```python
from build123d import *

# Parameters (mm, degrees)
SKETCH_1_W      = 99
SKETCH_1_H      = 29
EXTRUDE_2_DEPTH = 2
FILLET_1_R      = 2.5
SKETCH_3_W      = 103
SKETCH_3_H      = 33
EXTRUDE_3_DEPTH = 1
FILLET_2_R      = 0.2


with BuildPart() as part:
    # Эскиз1 → Бобышка-Вытянуть2 (new body)
    with BuildSketch(Plane.XY):
        with Locations((-70, 10)):
            Rectangle(SKETCH_1_W, SKETCH_1_H)
    extrude(amount=-EXTRUDE_2_DEPTH)

    # Скругление1
    fillet_1_edges = [part.edges().sort_by_distance(p)[0] for p in [
        (-119.5, 24.5, -1),
        (-20.5, 24.5, -1),
        (-20.5, -4.5, -1),
        (-119.5, -4.5, -1),
    ]]
    fillet(fillet_1_edges, radius=FILLET_1_R)

    # Эскиз3 → Бобышка-Вытянуть3 (add)
    with BuildSketch(Plane.XY.offset(-2)):
        with Locations((-70, 10)):
            Rectangle(SKETCH_3_W, SKETCH_3_H)
    extrude(amount=-EXTRUDE_3_DEPTH)

    # Скругление2
    fillet_2_edges = [part.edges().sort_by_distance(p)[0] for p in [
        (-70, -4.5, 0),
        (-119.5, 10, 0),
        (-20.5, 10, 0),
        (-70, 24.5, 0),
        (-21.232233047, 23.767766953, 0),
        (-118.767766953, 23.767766953, 0),
        (-118.767766953, -3.767766953, 0),
        (-21.232233047, -3.767766953, 0),
    ]]
    fillet(fillet_2_edges, radius=FILLET_2_R)


solid = part.part
```
Here's how the part is built. I have some questions about the finished solid (model axes, mm). A direction names the side the tool comes from. Coordinates: 2 decimals unless noted, no trailing zeros. Loops run counter-clockwise (first coordinate to the right, second up) from the corner with the lowest first, then second, coordinate; pieces in that order, holes last. Notation, with made-up numbers: M 68.5,-37.5 L 95.5,-37.5 A34 cw 95.5,-3.5 Z; hole C 52,-27 d4. An arc over 180 degrees is marked long. One line per item, written item: value.
1. Imagine slicing it at A-A (y = 16.5). List the corners of the cut face in (x, z) for me.
Geometry says:
outline: M -121.5,-3 L -18.5,-3 L -18.5,-2 L -20.5,-2 L -20.5,-0.2 A0.2 ccw -20.7,0 L -119.3,0 A0.2 ccw -119.5,-0.2 L -119.5,-2 L -121.5,-2 Z
2. Please list where these lines run through material, in increasing order: probe 1 along Y at (x, z) = (-61, -0.15); probe 2 along X at (y, z) = (20, -0.5).
Geometry says:
probe 1: y = -4.49 to 24.49
probe 2: x = -119.5 to -20.5
3. On a 3-axis mill with a long thin cutter (end or side, diameter ignored), from which of +Z, -Z, +X, -X, +Y, -Y can I reach the whole of each face in a straight line? I mean faces 1 (the flat face through (-71, 24.5, -1)), 2 (the flat face through (-119.5, 10, -1)), 3 (the cylindrical face through (-118.787, 23.748, -1.113)). Say none if no direction works.
Geometry says:
face 1: +Z, +X, -X, +Y
face 2: +Z, -X, +Y, -Y
face 3: +Z, -X, +Y
4. Will these pins go through, and if not, where does the flat tip stop? pin 1 Ø1.4 at (x, z) = (-65, -1) entering from -Y; pin 2 Ø0.5 at (x, z) = (-54.5, -1) entering from +Y; pin 3 Ø0.9 at (y, z) = (15, -1.5) entering from -X.
Geometry says:
pin 1: stops at y = -4.5
pin 2: stops at y = 24.5
pin 3: stops at x = -119.5
5. Imagine slicing it at B-B (z = -1.45). List the corners of the cut face in (x, y) for me, and give its area (3 significant figures).
Geometry says:
outline: M -119.5,-2 A2.5 ccw -117,-4.5 L -23,-4.5 A2.5 ccw -20.5,-2 L -20.5,22 A2.5 ccw -23,24.5 L -117,24.5 A2.5 ccw -119.5,22 Z
area: 2,870 mm2
6. Imagine slicing it at C-C (x = -68.5). List the corners of the cut face in (y, z) for me, and give its area (3 significant figures).
Geometry says:
outline: M -6.5,-3 L 26.5,-3 L 26.5,-2 L 24.5,-2 L 24.5,-0.2 A0.2 ccw 24.3,0 L -4.3,0 A0.2 ccw -4.5,-0.2 L -4.5,-2 L -6.5,-2 Z
area: 91.0 mm2
